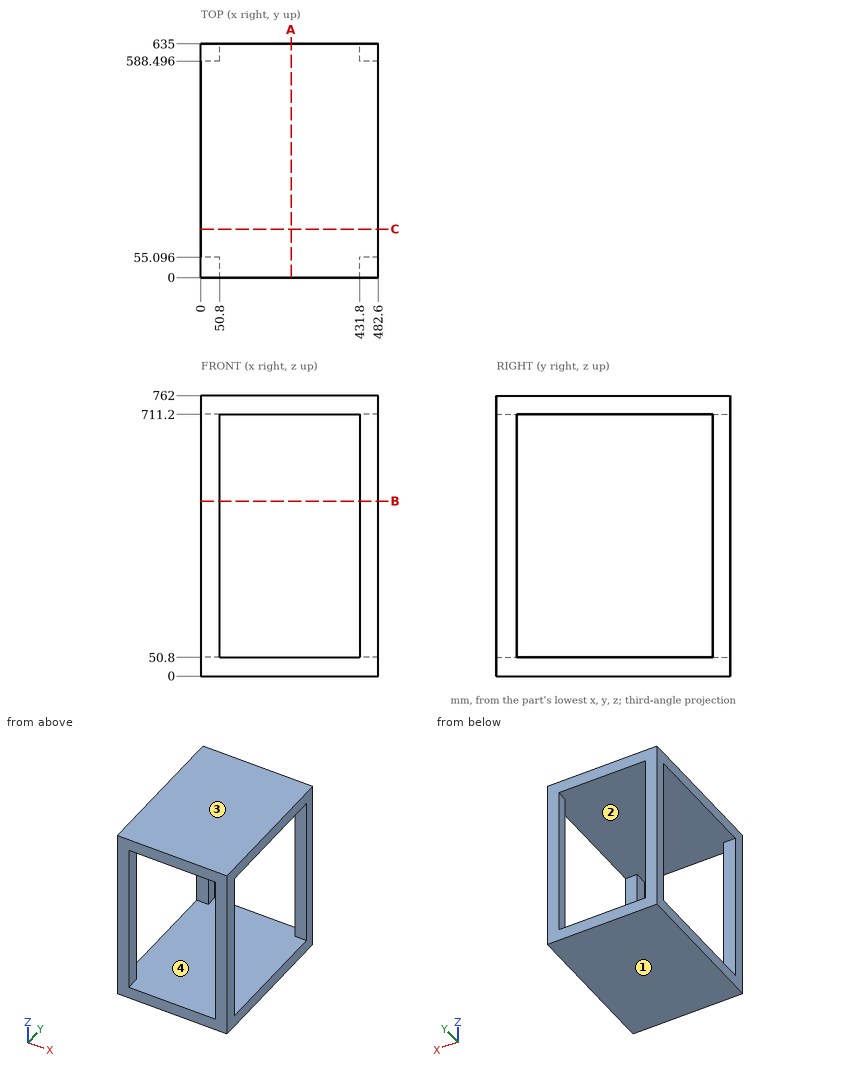
Answer from the drawing. Dimensions are ordinates in mm from the lowest x, y and z of the part. A direction names the side the tool comes from. Coordinates: 2 decimals unless noted, no trailing zeros. Write each loop counter-clockwise with the first axis right and the second up, starting at its lowest first coordinate (ties: lowest second). Pieces come first, ordered by that corner, then holes. Notation, with made-up numbers: (83, 40.5) - (96, 40.5) arc R29 ccw to (96, 69.5) - close; hole circle Ø2 at (40, 31). An arc over 180 degrees is marked (long way). Return JSON: item names as keys, results as strings.
1. The part is cut by section C-C on y = 132. Determine the outline of the cut face in (x, z), then the cut area to 3 significant figures.
Final values:
{"outline": "(0, 0) - (482.6, 0) - (482.6, 50.8) - (0, 50.8) - close; (0, 711.2) - (482.6, 711.2) - (482.6, 762) - (0, 762) - close", "area": "49,000 mm^2"}
2. This flat-tipped pin is pushed along its axis until it touches: pin 1 Ø16.5 at (y, z) = (36, 289) entering from -X. Where does it stop, or does it pass through?
Final values:
{"pin 1": "x = 0"}
3. The part is cut by section B-B on z = 475.5. Determine the outline of the cut face in (x, y), then the cut area to 3 significant figures.
Final values:
{"outline": "(0, 0) - (50.8, 0) - (50.8, 55.1) - (0, 55.1) - close; (0, 588.5) - (50.8, 588.5) - (50.8, 635) - (0, 635) - close; (431.8, 0) - (482.6, 0) - (482.6, 55.1) - (431.8, 55.1) - close; (431.8, 588.5) - (482.6, 588.5) - (482.6, 635) - (431.8, 635) - close", "area": "10,300 mm^2"}
4. Which of the six approach directions +Z, -Z, +X, -X, +Y, -Y give full straight-line access (tool end or side, diameter ignored) to the marked faces 3 and 4?
Final values:
{"face 3": "+Z, +X, -X, +Y, -Y", "face 4": "none"}
5. Consider line 1 along Z through (x, y) = (284, 353); line 2 along Y through (x, z) = (21.5, 204). Determine where each line is inside the solid, lowest interval first.
Final values:
{"line 1": "0 to 50.8, 711.2 to 762", "line 2": "0 to 55.1, 588.5 to 635"}
6. The part is cut by section A-A on x = 245. Determine the outline of the cut face in (y, z).
Final values:
{"outline": "(0, 0) - (635, 0) - (635, 50.8) - (0, 50.8) - close; (0, 711.2) - (635, 711.2) - (635, 762) - (0, 762) - close"}
7. For a pull along Y with two mould halves and no side action, classify the marked faces 1 and 2 as +Y half, -Y half, draft (parallel to the pull), parting line (faces both ways), or undercut.
Final values:
{"face 1": "draft", "face 2": "undercut"}
